Check sheet for the modelled part. Datum: model origin and axes. Units: mm. A direction names the side the tool comes from. Give positions to 0.01 mm unless a question says otherwise; leave off trailing zeros. Loops run counter-clockwise (first coordinate to the right, second up) from the corner with the lowest first, then second, coordinate; pieces in that order, holes last. Notation, with made-up numbers: (-12.75, -30) - (37.25, -30) arc R27 ccw to (37.25, -10) - close; hole circle Ø7 at (32.5, 84). An arc over 180 degrees is marked (long way). Use CSV: the item, a comma, the result in double quotes.
from build123d import *

# Parameters (mm, degrees)
BOSS_EXTRUDE1_DEPTH = 280
SKETCH3_R           = 2.5
CUT_EXTRUDE2_DEPTH  = 8
FILLET1_R           = 4
SKETCH4_R           = 5
CUT_EXTRUDE3_DEPTH  = 10


with BuildPart() as part:
    # Sketch1 → Boss-Extrude1 (new body)
    with BuildSketch(Plane(origin=(0, 0, 0), x_dir=(0, 0, -1), z_dir=(1, 0, 0))):
        Polygon((0, 0), (-60, 0), (-60, 24), (-40, 24), (-40, 44), (-20, 44), (-20, 24), (0, 24), align=None)
    extrude(amount=BOSS_EXTRUDE1_DEPTH)

    # Sketch3 → Cut-Extrude2 (cut)
    with BuildSketch(Plane(origin=(0, 24, 0), x_dir=(1, 0, 0), z_dir=(0, 1, 0))):
        with Locations(Location((115, -55, 0), (0, 0, 270))):
            Circle(SKETCH3_R)
        with Locations(Location((275, -55, 0), (0, 0, 270))):
            Circle(SKETCH3_R)
        with Locations(Location((275, -5, 0), (0, 0, 90))):
            Circle(SKETCH3_R)
        with Locations(Location((115, -5, 0), (0, 0, 90))):
            Circle(SKETCH3_R)
    extrude(amount=-CUT_EXTRUDE2_DEPTH, mode=Mode.SUBTRACT)

    # Fillet1
    fillet1_edges = [part.edges().sort_by_distance(p)[0] for p in [
        (140, 24, 40),
        (140, 24, 20),
    ]]
    fillet(fillet1_edges, radius=FILLET1_R)

    # Sketch4 → Cut-Extrude3 (cut)
    with BuildSketch(Plane(origin=(0, 44, 0), x_dir=(1, 0, 0), z_dir=(0, 1, 0))):
        with Locations(Location((20, -30, 0), (0, 0, 270))):
            Circle(SKETCH4_R)
    extrude(amount=-CUT_EXTRUDE3_DEPTH, mode=Mode.SUBTRACT)


solid = part.part
1. Sectioned sample at D-D, the plane x = 275. Record the boundary of the cut face in (y, z).
Completed:
outline,"(0, 0) - (24, 0) - (24, 2.5) - (16, 2.5) - (16, 7.5) - (24, 7.5) - (24, 16) arc R4 cw to (28, 20) - (44, 20) - (44, 40) - (28, 40) arc R4 cw to (24, 44) - (24, 52.5) - (16, 52.5) - (16, 57.5) - (24, 57.5) - (24, 60) - (0, 60) - close"
2. Release check for a two-part mould opening along Z. For faces 1 (the face through (117.48, 20.06, 54.67)), 2 (the face through (138, 12, 0)), 3 (the face through (138, 24, 52)) record: released by +Z, released by -Z, zero draft, split by the parting line, or undercut.
Completed:
face 1,"undercut"
face 2,"released by -Z"
face 3,"zero draft"
3. Sectioned sample at A-A, the plane z = 5. Record the boundary of the cut face in (x, y).
Completed:
outline,"(0, 0) - (280, 0) - (280, 24) - (277.5, 24) - (277.5, 16) - (272.5, 16) - (272.5, 24) - (117.5, 24) - (117.5, 16) - (112.5, 16) - (112.5, 24) - (0, 24) - close"
4. Go/stop test with flat-tipped pins: pin 1 Ø6 at (x, z) = (20, 30) entering from +Y; pin 2 Ø8 at (x, z) = (163, 51.5) entering from +Y; pin 3 Ø2.5 at (x, z) = (114.5, 55) entering from +Y. Record where each tip stops, or that it passes through.
Completed:
pin 1,"stops at y = 34"
pin 2,"stops at y = 24"
pin 3,"stops at y = 16"
5. Set-up check for faces 4 (the face through (275, 16, 5)), 5 (the face through (138, 24, 8)), 6 (the face through (138, 36, 40)), 7 (the face through (0, 17, 30)), 8 (the face through (280, 17, 30)): record each of +Z, -Z, +X, -X, +Y, -Y from which the full face is reachable in a straight line by a thin tool's end or side.
Completed:
face 4,"+Y"
face 5,"-Z, +X, -X, +Y"
face 6,"+Z, +X, -X, +Y"
face 7,"+Z, -Z, -X, +Y, -Y"
face 8,"+Z, -Z, +X, +Y, -Y"
6. Sectioned sample at C-C, the plane y = 31.5. Record the boundary of the cut face in (x, z), and give its area (3 significant figures).
Completed:
outline,"(0, 20) - (280, 20) - (280, 40) - (0, 40) - close"
area,"5,600 mm²"
7. Sectioned sample at B-B, the plane x = 20. Record the boundary of the cut face in (y, z).
Completed:
outline,"(0, 0) - (24, 0) - (24, 16) arc R4 cw to (28, 20) - (44, 20) - (44, 25) - (34, 25) - (34, 35) - (44, 35) - (44, 40) - (28, 40) arc R4 cw to (24, 44) - (24, 60) - (0, 60) - close"
8. Scan lines: line 1 along X through (y, z) = (21.5, 5); line 2 along X through (y, z) = (37.25, 30); line 3 along Y through (x, z) = (65, 3.5). Record each from-to range of solid material in increasing order.
Completed:
line 1,"x = 0 to 112.5, 117.5 to 272.5, 277.5 to 280"
line 2,"x = 0 to 15, 25 to 280"
line 3,"y = 0 to 24"
